Geometry: final body of the model. Coordinates: model frame, mm. A direction names the side the tool comes from. Give positions to 0.01 mm unless a question says otherwise; leave off trailing zeros. Order: outer loops, then holes, each group sorted by start corner. A loop starts at its lowest first (then second) coordinate and runs counter-clockwise, first axis right, second up. Notation, with made-up numbers: (57.5, 62) - (79.5, 62) arc R23 ccw to (79.5, 81) - close; hole circle Ø7 at (53, -8). An arc over 180 degrees is marked (long way). Use one line per item in the form item = value.
from build123d import *

# Parameters (mm, degrees)
SKETCH1_W                 = 83
SKETCH1_H                 = 100
BOSS_EXTRUDE1_DEPTH       = 1.5875
F_0_CLEARANCE_HOLE1_D     = 1.778
F_0_CLEARANCE_HOLE1_DEPTH = 3.175
F_0_CLEARANCE_HOLE1_TIP   = 0.53416509
SKETCH5_W                 = 50
SKETCH5_H                 = 16.6
BOSS_EXTRUDE3_DEPTH       = 0.1
SKETCH6_W                 = 55
SKETCH6_H                 = 5
BOSS_EXTRUDE4_DEPTH       = 0.1
SKETCH7_W                 = 4.99
SKETCH7_H                 = 5
BOSS_EXTRUDE5_DEPTH       = 0.1


with BuildPart() as part:
    # Sketch1 → Boss-Extrude1 (new body)
    with BuildSketch(Plane.XY):
        Rectangle(SKETCH1_W, SKETCH1_H)
    extrude(amount=BOSS_EXTRUDE1_DEPTH)

    # #0 Clearance Hole1
    with Locations(Plane.XY.offset(1.5875)):
        with Locations((-39, 42.5), (-39, 22.5), (-39, 2.5), (-39, -17.5), (-39, -37.5), (39, -37.5), (39, -17.5), (39, 2.5), (39, 22.5), (39, 42.5)):
            Hole(F_0_CLEARANCE_HOLE1_D / 2, depth=F_0_CLEARANCE_HOLE1_DEPTH)
            with Locations((0, 0, -(F_0_CLEARANCE_HOLE1_DEPTH + F_0_CLEARANCE_HOLE1_TIP / 2))):  # 118° drill point
                Cone(0, F_0_CLEARANCE_HOLE1_D / 2, F_0_CLEARANCE_HOLE1_TIP, mode=Mode.SUBTRACT)

    # Sketch5 → Boss-Extrude3 (add)
    with BuildSketch(Plane.XY.offset(1.5875)):
        with Locations((0, 14.6)):
            Rectangle(SKETCH5_W, SKETCH5_H)
        with Locations((0, 31.7)):
            Rectangle(SKETCH5_W, SKETCH5_H)
        with Locations((0, -2.5)):
            Rectangle(SKETCH5_W, SKETCH5_H)
        with Locations((0, -19.6)):
            Rectangle(SKETCH5_W, SKETCH5_H)
        with Locations((0, -36.7)):
            Rectangle(SKETCH5_W, SKETCH5_H)
    extrude(amount=BOSS_EXTRUDE3_DEPTH)

    # Sketch6 → Boss-Extrude4 (add)
    with BuildSketch(Plane.XY.offset(1.5875)):
        with Locations((2.5, 42.6)):
            Rectangle(SKETCH6_W, SKETCH6_H)
    extrude(amount=BOSS_EXTRUDE4_DEPTH)

    # Sketch7 → Boss-Extrude5 (add)
    with BuildSketch(Plane.XY.offset(1.5875)):
        with Locations((27.505, -42.5)):
            Rectangle(SKETCH7_W, SKETCH7_H)
    extrude(amount=BOSS_EXTRUDE5_DEPTH)


solid = part.part
(1) Contact query for flat-ended pins moving along their axis: pin 1 Ø10 at (x, y) = (-13.5, -33) entering from -Z; pin 2 Ø1.6 at (x, y) = (-39, 42.5) entering from +Z; pin 3 Ø2 at (x, y) = (39, 2.5) entering from +Z. Output: stop coordinate, or through.
Computed values:
pin_1 = 0
pin_2 = through
pin_3 = 1.59
(2) Ray query, line 1 along Y through (x, z) = (-39, 1); line 2 along X through (y, z) = (-37.5, 0.9); line 3 along Z through (x, y) = (29, -26). Return the intervals inside material, ascending.
Computed values:
line_1 = -50 to -38.39, -36.61 to -18.39, -16.61 to 1.61, 3.39 to 21.61, 23.39 to 41.61, 43.39 to 50
line_2 = -41.5 to -39.89, -38.11 to 38.11, 39.89 to 41.5
line_3 = 0 to 1.59
(3) Reachability of faces 1 (the face through (-28, 12, 1.588)), 2 (the face through (27, -42, 1.688)) from +Z, -Z, +X, -X, +Y, -Y: full face, straight path, thin tool, end or side. Return the list, or none.
Computed values:
face_1 = +Z
face_2 = +Z, +X, -X, +Y, -Y
(4) Cut plane A-A on y = 37.5. Output: boundary loops of the cut face in (x, z).
Computed values:
outline = (-41.5, 0) - (41.5, 0) - (41.5, 1.59) - (25, 1.59) - (25, 1.69) - (-25, 1.69) - (-25, 1.59) - (-41.5, 1.59) - close
